CAD build for the part. Positions are in the model's coordinates, mm. Face numbers are marked on the shaded views. Coordinates: 2 decimals unless noted, no trailing zeros. Order: outer loops, then holes, each group sorted by start corner. A loop starts at its lowest first (then second) coordinate and runs counter-clockwise, first axis right, second up. Notation, with made-up numbers: M 51.25,7 L 60.25,7 A23 cw 60.25,34 Z; hole C -5,-7 d3. An arc over 180 degrees is marked long. Write item = value, one per line. Start each with the question number.
```python
from build123d import *

# Parameters (mm, degrees)
F0_W     = 150
F0_H     = 50
F1_DEPTH = 12
F2_D     = 10


with BuildPart() as f1:
    # F0 (on Front) → F1 (new body)
    with BuildSketch(Plane.XZ):
        Rectangle(F0_W, F0_H)
    extrude(amount=-F1_DEPTH)

    # F2 (through all)
    with Locations(Plane.XZ):
        with Locations((-49, -3), (49, -3)):
            Hole(F2_D / 2)


solid = f1.part
```
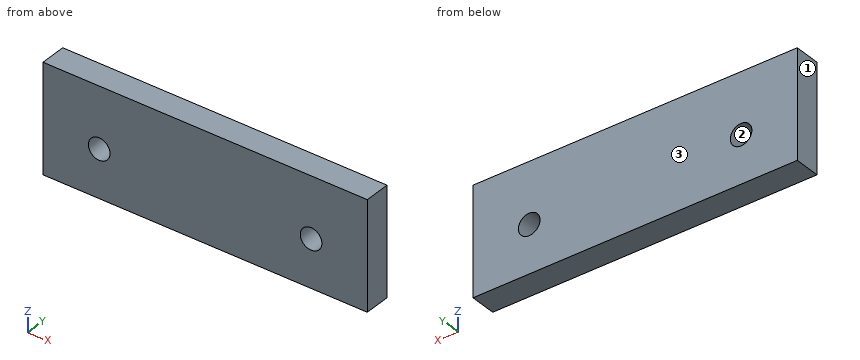
1. Slice it at C-C (y = 9.25). Write the cut outline in (x, z), plus the area to 3 significant figures.
2. Slice it at B-B (z = -3). Write the cut outline in (x, y).
3. Slice it at A-A (x = -49). Write the cut outline in (y, z).
4. Probe L1, parallel to Z at x = -49, y = 3.25; L2, parallel to Z at x = 47.5, y = 4.75; L3, parallel to X at y = 8.25, z = -5. List the from-to ranges inside material, lowest first.
5. Flat gauge pins, fed straight in: pin 1 (11.5 mm diameter, centred on x = 49, z = -3, fed in from +Y); pin 2 (6 mm diameter, centred on x = -49, z = -3, fed in from -Y). Where does each tip first touch, or does it go through?
6. Mould opens along X. For the marked faces 1, 2 and 3 say: released by +X, released by -X, zero draft, split by the parting line, or undercut.
Calculated:
q1.outline = M -75,-25 L 75,-25 L 75,25 L -75,25 Z; hole C -49,-3 d10; hole C 49,-3 d10
q1.area = 7,340 mm²
q2.outline = M -75,0 L -54,0 L -54,12 L -75,12 Z; M -44,0 L 44,0 L 44,12 L -44,12 Z; M 54,0 L 75,0 L 75,12 L 54,12 Z
q3.outline = M 0,-25 L 12,-25 L 12,-8 L 0,-8 Z; M 0,2 L 12,2 L 12,25 L 0,25 Z
q4.L1 = -25 to -8, 2 to 25
q4.L2 = -25 to -7.77, 1.77 to 25
q4.L3 = -75 to -53.58, -44.42 to 44.42, 53.58 to 75
q5.pin_1 = 12
q5.pin_2 = through
q6.face_1 = released by -X
q6.face_2 = undercut
q6.face_3 = zero draft
